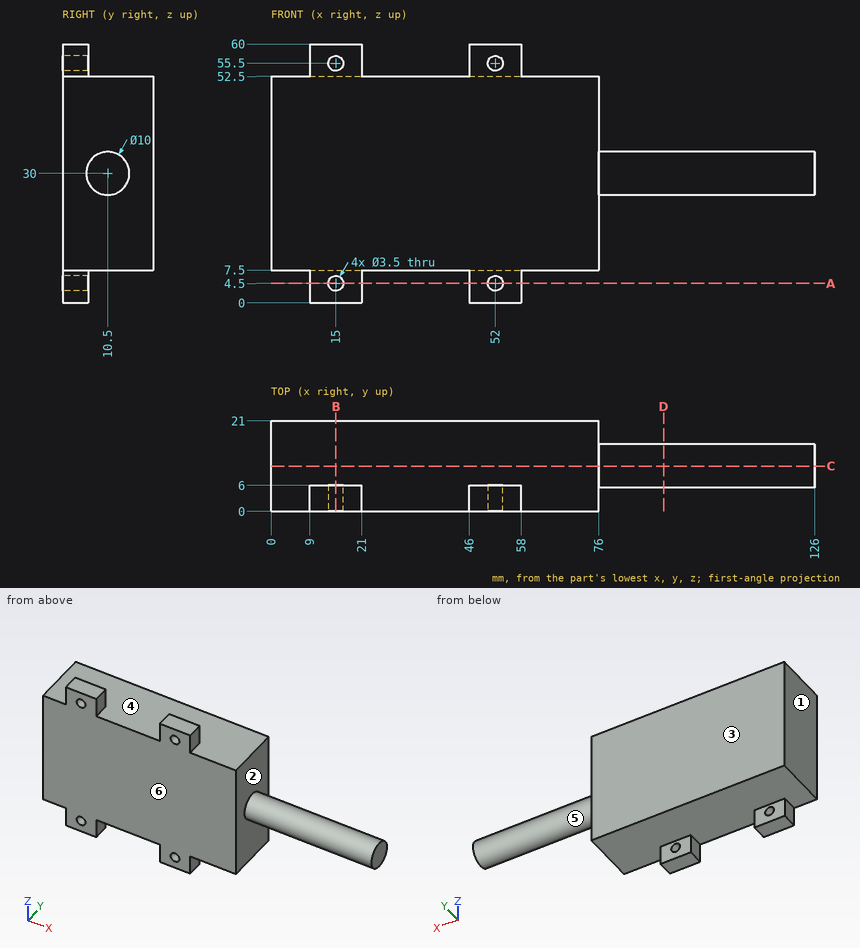
Can you work these out from the drawing? Everything is in mm from the part's minimum corner. A direction names the side the tool comes from. Give positions to 0.01 mm unless a question says otherwise; leave off trailing zeros. Order: outer loops, then holes, each group sorted by start corner. A loop starts at its lowest first (then second) coordinate and runs counter-clockwise, first axis right, second up. Notation, with made-up numbers: M 82.5,-29.5 L 129.5,-29.5 A31 cw 129.5,3.5 Z; hole C -30.75,70.25 d7. An arc over 180 degrees is marked long. Use a Markdown table: item, result. Add a question column.
1. Suppose I cut it at B-B (x = 15). List the corners of the cut face in (y, z) for me, and give its area (3 significant figures).
2. Suppose I cut it at D-D (x = 91). List the corners of the cut face in (y, z) for me, and give its area (3 significant figures).
3. Suppose I cut it at C-C (y = 10.5). List the corners of the cut face in (x, z) for me, and give its area (3 significant figures).
4. On a 3-axis mill with a long thin cutter (end or side, diameter ignored), from which of +Z, -Z, +X, -X, +Y, -Y can I reach the whole of each face in a straight line? I mean the marked faces 5 and 6. Say none if no direction works.
5. I need wall thicknesses on probe 1 along X at (y, z) = (1.65, 55.5); probe 2 along Z at (x, y) = (52, 3.4); probe 3 along X at (y, z) = (5.5, 3). Which ranges of each line are inside material? Lowest first, please. Write a range as from..to.
6. Suppose I cut it at A-A (z = 4.5). List the corners of the cut face in (x, y) for me, and give its area (3 significant figures).
7. If we mould it in two halves opening along X, with no side actions, what happens to the marked faces 1, 2, 3 and 4? For each: +X half, -X half, draft (parallel to the pull), parting line (faces both ways), or undercut.
8. For pin 1 Ø4.5 at (x, z) = (15, 4.5) entering from +Y; pin 2 Ø5 at (y, z) = (3, 4.5) entering from +X; pin 3 Ø3 at (y, z) = (3, 2.5) entering from -X, each with a flat end and sliding along its axis, tell me the tip position at first contact or that it passes through.
Results list:
| question | item | result |
|---|---|---|
| 1 | outline | M 0,0 L 6,0 L 6,2.75 L 0,2.75 Z; M 0,6.25 L 6,6.25 L 6,7.5 L 21,7.5 L 21,52.5 L 6,52.5 L 6,53.75 L 0,53.75 Z; M 0,57.25 L 6,57.25 L 6,60 L 0,60 Z |
| 1 | area | 993 mm² |
| 2 | outline | C 10.5,30 d10 |
| 2 | area | 78.5 mm² |
| 3 | outline | M 0,7.5 L 76,7.5 L 76,25 L 126,25 L 126,35 L 76,35 L 76,52.5 L 0,52.5 Z |
| 3 | area | 3,920 mm² |
| 4 | face 5 | +X |
| 4 | face 6 | +Z, -Z, +X, -X, -Y |
| 5 | probe 1 | x = 9..13.25, 16.75..21, 46..50.25, 53.75..58 |
| 5 | probe 2 | z = 0..2.75, 6.25..53.75, 57.25..60 |
| 5 | probe 3 | x = 9..14.1, 15.9..21, 46..51.1, 52.9..58 |
| 6 | outline | M 9,0 L 13.25,0 L 13.25,6 L 9,6 Z; M 16.75,0 L 21,0 L 21,6 L 16.75,6 Z; M 46,0 L 50.25,0 L 50.25,6 L 46,6 Z; M 53.75,0 L 58,0 L 58,6 L 53.75,6 Z |
| 6 | area | 102 mm² |
| 7 | face 1 | -X half |
| 7 | face 2 | +X half |
| 7 | face 3 | draft |
| 7 | face 4 | undercut |
| 8 | pin 1 | stops at y = 6 |
| 8 | pin 2 | stops at x = 58 |
| 8 | pin 3 | stops at x = 9 |
